```python
from build123d import *

# Parameters (mm, degrees)
SKETCH_1_W               = 150
SKETCH_1_H               = 100
EXTRUDE_1_DEPTH          = 0.5
CUT_EXTRUDE_1_DEPTH      = 91.140168626
CUT_EXTRUDE_1_DEPTH_BACK = 91.140168626
SKETCH_2_R               = 1.5


with BuildPart() as part:
    # 草图1 → 凸台-拉伸1 (new, symmetric)
    with BuildSketch(Plane(origin=(0, 0, 0), x_dir=(1, 0, 0), z_dir=(0, 1, 0))):
        Rectangle(SKETCH_1_W, SKETCH_1_H)
    extrude(amount=EXTRUDE_1_DEPTH, both=True)

    # 草图2 → 切除-拉伸1 (cut, two sides: drawn at the far end of the back side and taken through both)
    with BuildSketch(Plane(origin=(0, 0, 0), x_dir=(1, 0, 0), z_dir=(0, 1, 0)).offset(-CUT_EXTRUDE_1_DEPTH_BACK)):
        with Locations(Location((-70.75, 45, 0), (0, 0, 270))):
            Circle(SKETCH_2_R)
        with Locations(Location((70.75, 45, 0), (0, 0, 270))):
            Circle(SKETCH_2_R)
        with Locations(Location((-70.75, -45, 0), (0, 0, 270))):
            Circle(SKETCH_2_R)
        with Locations(Location((70.75, -45, 0), (0, 0, 270))):
            Circle(SKETCH_2_R)
    extrude(amount=CUT_EXTRUDE_1_DEPTH + CUT_EXTRUDE_1_DEPTH_BACK, mode=Mode.SUBTRACT)


solid = part.part
```
The model under review builds one solid part; all positions refer to its coordinate system, in mm. Round coordinates to 2 decimals unless told otherwise and drop trailing zeros. Order: outer loops, then holes, each group sorted by start corner. A loop starts at its lowest first (then second) coordinate and runs counter-clockwise, first axis right, second up.
Item 1: For pin 1 (2.5 mm diameter, centred on x = -70.75, z = -45, fed in from +Y) (3 decimals), flat-tipped, find the tip position at first contact; note if it passes through.
Working result:
pin 1: passes through
Item 2: Add section B-B, the plane x = 70.75. State the section outline as (y, z) points, and give its area (3 significant figures).
Working result:
outline: (-0.5, -50) - (0.5, -50) - (0.5, -46.5) - (-0.5, -46.5) - close; (-0.5, -43.5) - (0.5, -43.5) - (0.5, 43.5) - (-0.5, 43.5) - close; (-0.5, 46.5) - (0.5, 46.5) - (0.5, 50) - (-0.5, 50) - close
area: 94.0 mm2
Item 3: To check wall thickness, follow probe 1 along Z at (x, y) = (-70.75, -0.3); probe 2 along X at (y, z) = (0, -45). State the ranges of each line that lie inside material, in increasing order.
Working result:
probe 1: z = -50 to -46.5, -43.5 to 43.5, 46.5 to 50
probe 2: x = -75 to -72.25, -69.25 to 69.25, 72.25 to 75
Item 4: Draft analysis for pull direction X (two halves, no side actions). For faces 1 (the flat face through (-1, 0.5, -1)), 2 (the cylindrical face through (-70.7, 0, -46.5)), state which applies: released by +X, released by -X, zero draft, split by the parting line, or undercut.
Working result:
face 1: zero draft
face 2: undercut
Item 5: Add section A-A, the plane z = -45. State the section outline as (x, y) points.
Working result:
outline: (-75, -0.5) - (-72.25, -0.5) - (-72.25, 0.5) - (-75, 0.5) - close; (-69.25, -0.5) - (69.25, -0.5) - (69.25, 0.5) - (-69.25, 0.5) - close; (72.25, -0.5) - (75, -0.5) - (75, 0.5) - (72.25, 0.5) - close
